Design review of the part built by this model. Coordinates are the model's own, in mm. A direction names the side the tool comes from. Round coordinates to 2 decimals unless told otherwise and drop trailing zeros. Order: outer loops, then holes, each group sorted by start corner. A loop starts at its lowest first (then second) coordinate and runs counter-clockwise, first axis right, second up. Notation, with made-up numbers: M 82.25,-14 L 139.25,-14 A26 cw 139.25,25 Z; hole C -32.5,-18.75 d7. An arc over 180 degrees is marked long. Use a Markdown table: item, result. Add a question column.
(1) Take a section at D-D (y = 2.5). Write out the cut boundary in (x, z).
(2) The part is to be moulded in two halves that separate along Z. For faces 1 (the face through (14.41, 0.79, 26.94)), 2 (the face through (13.51, 6, 10)), 3 (the face through (-20.725, 0.811, 19.578)), say which applies: released by +Z, released by -Z, zero draft, split by the parting line, or undercut.
(3) To check wall thickness, follow probe 1 along X at (y, z) = (0.8, 19.35); probe 2 along Y at (x, z) = (-13, 4); probe 3 along X at (y, z) = (5, 1.5). State the ranges of each line that lie inside material, in increasing order. Write a range as from..to.
(4) Machinability: for faces 4 (the face through (14, 6, 0.69)), 5 (the face through (12, 6, 8.5)), 6 (the face through (16.11, 6, 6)), 7 (the face through (-25.26, 0.79, 15.74)), 8 (the face through (10.91, 6, 5)), which of the approach directions +Z, -Z, +X, -X, +Y, -Y give a long, thin tool a straight path to every point of the face, cutting with its end or side? Answer none if there is none.
(5) Take a section at A-A (z = 19.5). Write out the cut boundary in (x, y), then the cut area to 3 significant figures.
(6) Take a section at C-C (z = -26.5). Write out the cut boundary in (x, y).
(7) Take a section at B-B (x = 20). Write out the cut boundary in (y, z).
(8) For pin 1 (4 mm diameter, centred on x = 13.5, y = 4.5, fed in from -Z); pin 2 (1.5 mm diameter, centred on y = 7.5, z = 9.5, fed in from +X); pin 3 (2 mm diameter, centred on y = 1, z = -16, fed in from +X), all flat-tipped, find the tip position at first contact; note any pin that passes through.
```python
from build123d import *

# Parameters (mm, degrees)
BOSS_EXTRUDE1_DEPTH = 1.6
SKETCH2_R           = 1.75
CUT_EXTRUDE1_DEPTH  = 1.6
BOSS_EXTRUDE2_DEPTH = 9


with BuildPart() as part:
    # Sketch1 → Boss-Extrude1 (new body)
    with BuildSketch(Plane(origin=(0, 0, 0), x_dir=(1, 0, 0), z_dir=(0, 1, 0))):
        Polygon((0, 31.15), (22.4, 22.15), (28.2, 7.75), (28.2, -8.44), (22.4, -22.84), (6.2, -31.15), (-6.2, -31.15), (-22.4, -22.84), (-28.2, -8.44), (-28.2, 7.75), (-22.4, 22.15), align=None)
    extrude(amount=BOSS_EXTRUDE1_DEPTH)

    # Sketch2 → Cut-Extrude1 (cut)
    with BuildSketch(Plane(origin=(0, 1.6, 0), x_dir=(1, 0, 0), z_dir=(0, 1, 0))):
        with Locations(Location((0, 26.28, 0), (0, 0, 270))):
            Circle(SKETCH2_R)
        with Locations(Location((18.99, -19.35, 0), (0, 0, 270))):
            Circle(SKETCH2_R)
        with Locations(Location((-18.99, -19.35, 0), (0, 0, 90))):
            Circle(SKETCH2_R)
    extrude(amount=-CUT_EXTRUDE1_DEPTH, mode=Mode.SUBTRACT)

    # Sketch3 → Boss-Extrude2 (add)
    with BuildSketch(Plane(origin=(0, 1.6, 0), x_dir=(1, 0, 0), z_dir=(0, 1, 0))):
        Polygon((13.51, -8.5), (13.51, -11.05), (16.11, -11.05), (16.11, -0.69), (13.51, -0.69), (10.91, -0.69), (10.91, -8.5), align=None)
    extrude(amount=BOSS_EXTRUDE2_DEPTH)


solid = part.part
```
Verdict:
| question | item | result |
|---|---|---|
| 1 | outline | M 10.91,0.69 L 16.11,0.69 L 16.11,11.05 L 13.51,11.05 L 13.51,8.5 L 10.91,8.5 Z |
| 2 | face 1 | released by +Z |
| 2 | face 2 | zero draft |
| 2 | face 3 | undercut |
| 3 | probe 1 | x = -23.81..-20.74, -17.24..17.24, 20.74..23.81 |
| 3 | probe 2 | y = 0..1.6 |
| 3 | probe 3 | x = 10.91..16.11 |
| 4 | face 4 | -Z, +X, -X, +Y |
| 4 | face 5 | +Z, -X, +Y |
| 4 | face 6 | +Z, -Z, +X, +Y |
| 4 | face 7 | +Z, -X, +Y, -Y |
| 4 | face 8 | +Z, -Z, -X, +Y |
| 5 | outline | M -23.75,0 L -20.73,0 L -20.73,1.6 L -23.75,1.6 Z; M -17.25,0 L 17.25,0 L 17.25,1.6 L -17.25,1.6 Z; M 20.73,0 L 23.75,0 L 23.75,1.6 L 20.73,1.6 Z |
| 5 | area | 64.8 mm^2 |
| 6 | outline | M -11.57,0 L -1.74,0 L -1.74,1.6 L -11.57,1.6 Z; M 1.74,0 L 11.57,0 L 11.57,1.6 L 1.74,1.6 Z |
| 7 | outline | M 0,-23.11 L 1.6,-23.11 L 1.6,17.92 L 0,17.92 Z; M 0,20.78 L 1.6,20.78 L 1.6,24.07 L 0,24.07 Z |
| 8 | pin 1 | stops at z = 0.69 |
| 8 | pin 2 | stops at x = 16.11 |
| 8 | pin 3 | stops at x = 25.28 |
